Check sheet for the modelled part. Datum: model origin and axes. Units: mm. A direction names the side the tool comes from. Round coordinates to 2 decimals unless told otherwise and drop trailing zeros. Write each loop counter-clockwise with the first axis right and the second up, starting at its lowest first coordinate (ties: lowest second). Pieces come first, ordered by that corner, then holes.
Item 1: Go/stop test with flat-tipped pins: pin 1 Ø6 at (y, z) = (4.5, -1.5) entering from +X; pin 2 Ø10 at (x, y) = (2044.5, 4.5) entering from -Z; pin 3 Ø10 at (y, z) = (5.5, 1) entering from +X; pin 4 Ø3 at (x, z) = (2053, -19.5) entering from -Y. Record where each tip stops, or that it passes through.
Item 2: Cross-section at B-B on z = -13.5. Enter the section's corners in (x, y).
Item 3: Material ranges on line 1 (X direction, y = 3.5, z = -22); line 2 (X direction, y = 11.25, z = -3.5); line 3 (Z direction, x = 2028, y = 21), recorded low to high.
Item 4: Tool access check on faces 4 (the flat face through (2032, 13, -25.248)), 5 (the cylindrical face through (2054.76, 12.52, -20.89)), 6 (the flat face through (2062.15, 12.52, -4.63)). Record the directions out of +Z, -Z, +X, -X, +Y, -Y that give a thin tool (end or side, any length) a straight path to the whole face; none if there is none.
Item 5: Cross-section at A-A on y = 21.75. Enter the section's corners in (x, z), plus the area to 3 significant figures.
Item 6: Release check for a two-part mould opening along Z. For faces 1 (the flat face through (2060.6, 12.5, 8.3)), 2 (the flat face through (2038.212, 13, -26)), 3 (the flat face through (2061.83, 12.52, 1.7)) record: +Z half, -Z half, draft (parallel to the pull), parting line (faces both ways), or undercut.
Item 7: Cross-section at C-C on x = 2029.5. Enter the section's corners in (y, z).
Autodesk Fusion 360 part; units mm, degrees
sketch "Front, Bottom corner" plane through (0, 0, 0) normal (0, 1, 0) x (1, 0, 0)
  circle A0 centre (2038.212, 2.1526) radius 25 construction
  line L0 (2073.9927, -100.7451) -> (2060.9213, 25.5804) construction
  line L1 (1557.274, 27.1526) -> (2059.178, 27.1526) construction
  line L2 (2038.212, 27.1526) -> (2038.212, 25.2476)
  line L3 (2038.212, 25.2476) -> (2025.512, 25.2476)
  line L4 (2025.512, 25.2476) -> (2025.512, 21.4376)
  line L5 (2063.0792, 4.7257) -> (2061.1843, 4.5296)
  line L6 (2061.1843, 4.5296) -> (2062.4914, -8.1029)
  line L7 (2062.4914, -8.1029) -> (2058.7017, -8.4951)
  arc A1 (2063.0792, 4.7257) -> (2038.212, 27.1526) centre (2038.212, 2.1526) ccw
  line L8 (2038.212, 2.1526) -> (2054.9552, 20.7177) construction
  arc A2 (2058.7017, -8.4951) -> (2025.512, 21.4376) centre (2030.3296, -6.5875) ccw
  point P0 (2049.3741, 14.5294)
extrude "Extrude1" add sketch "Front, Bottom corner" along normal blind 25.4
Response values:
1. pin 1: stops at x = 2061.81
1. pin 2: stops at z = -27.12
1. pin 3: stops at x = 2062.27
1. pin 4: stops at y = 0
2. outline: (2050.46, 0) - (2060.49, 0) - (2060.49, 25.4) - (2050.46, 25.4) - close
3. line 1: x = 2025.51 to 2053.41
3. line 2: x = 2056.92 to 2061.29
3. line 3: z = -25.25 to -21.75
4. face 4: -Z, -X, +Y, -Y
4. face 5: -Z, +X, +Y, -Y
4. face 6: +X, +Y, -Y
5. outline: (2025.51, -25.25) - (2038.21, -25.25) - (2038.21, -27.15) arc R25 ccw to (2063.08, -4.73) - (2061.18, -4.53) - (2062.49, 8.1) - (2058.7, 8.5) arc R28.44 cw to (2025.51, -21.44) - close
5. area: 332 mm2
6. face 1: +Z half
6. face 2: draft
6. face 3: undercut
7. outline: (0, -25.25) - (25.4, -25.25) - (25.4, -21.84) - (0, -21.84) - close
